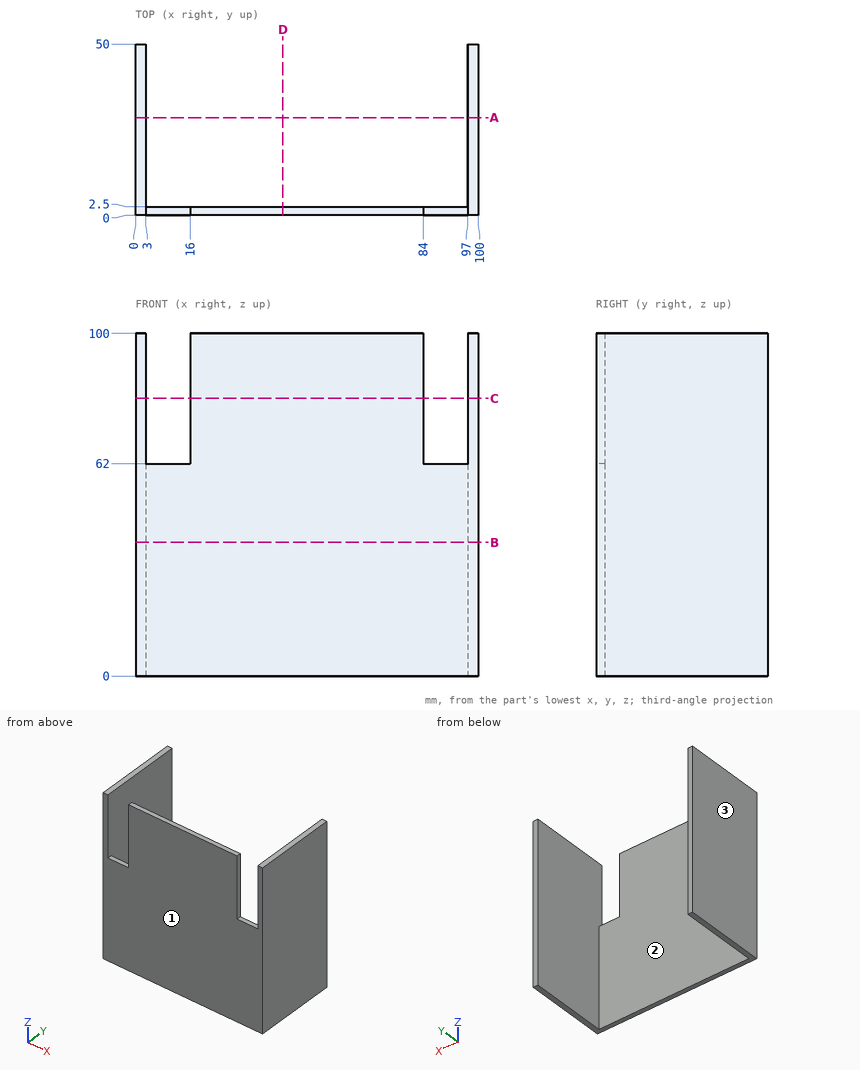
Answer from the drawing. Dimensions are ordinates in mm from the lowest x, y and z of the part. Round coordinates to 2 decimals unless told otherwise and drop trailing zeros. Write each loop counter-clockwise with the first axis right and the second up, starting at its lowest first coordinate (ties: lowest second). Pieces come first, ordered by that corner, then holes. Notation, with made-up numbers: M -30.5,30 L 17.5,30 A12 cw 17.5,40 Z; hole C -5.75,25 d9. An arc over 180 degrees is marked long. Write each question's results on one line, items separated by ' | '. Start each with the question number.
Item 1: The mould has two halves that part along X. Classify the marked faces 1, 2 and 3: +X half, -X half, draft (parallel to the pull), parting line (faces both ways), or undercut.
Item 2: Find section D-D on x = 43. Write down the section's boundary in (y, z).
Item 3: Find section B-B on z = 39. Write down the section's boundary in (x, y), and give its area (3 significant figures).
Item 4: Find section A-A on y = 28.5. Write down the section's boundary in (x, z).
Item 5: Straight lines are drawn through the part: probe 1 along X at (y, z) = (32.5, 70.5); probe 2 along Y at (x, z) = (27, 68.5). For each, find the intervals that lie inside material, in ascending order.
Item 6: Given pin 1 Ø3 at (x, y) = (8.5, 1.5) entering from +Z; pin 2 Ø12 at (x, z) = (22, 57) entering from +Y, each flat-ended and moving along its own axis, determine where each tip first touches the part or whether it passes through.
Item 7: Find section C-C on z = 81. Write down the section's boundary in (x, y).
Answer block:
1) face 1: draft | face 2: undercut | face 3: -X half
2) outline: M 0,0 L 2.5,0 L 2.5,100 L 0,100 Z
3) outline: M 0,0 L 100,0 L 100,50 L 97,50 L 97,2.5 L 3,2.5 L 3,50 L 0,50 Z | area: 535 mm²
4) outline: M 0,0 L 3,0 L 3,100 L 0,100 Z; M 97,0 L 100,0 L 100,100 L 97,100 Z
5) probe 1: x = 0 to 3, 97 to 100 | probe 2: y = 0 to 2.5
6) pin 1: stops at z = 62 | pin 2: stops at y = 2.5
7) outline: M 0,0 L 3,0 L 3,50 L 0,50 Z; M 16,0 L 84,0 L 84,2.5 L 16,2.5 Z; M 97,0 L 100,0 L 100,50 L 97,50 Z
